CAD build for the part. Positions are in the model's coordinates, mm. A direction names the side the tool comes from. Coordinates: 2 decimals unless noted, no trailing zeros. Write each loop counter-clockwise with the first axis right and the second up, starting at its lowest first coordinate (ties: lowest second). Pieces come first, ordered by that corner, then holes. Notation, with made-up numbers: (-38.5, -20.5) -> (-9.5, -20.5) arc R22 cw to (-9.5, -8.5) -> close; hole circle Ø2 at (-25.75, 49.25). An arc over 180 degrees is marked (long way). Answer as CSV lines item,"result".
```python
from build123d import *

# Parameters (mm, degrees)
SKETCH1_W           = 12.7
SKETCH1_H           = 2.54
SKETCH1_W_2         = 1.27
SKETCH1_H_2         = 1.27
BOSS_EXTRUDE1_DEPTH = 2.54


with BuildPart() as part:
    # Sketch1 → Boss-Extrude1 (new body)
    with BuildSketch(Plane(origin=(0, 0, 0), x_dir=(1, 0, 0), z_dir=(0, 1, 0))):
        with Locations((6.35, 1.27)):
            Rectangle(SKETCH1_W, SKETCH1_H)
        with Locations((3.81, 1.27)):
            Rectangle(SKETCH1_W_2, SKETCH1_H_2, mode=Mode.SUBTRACT)
        with Locations((1.27, 1.27)):
            Rectangle(SKETCH1_W_2, SKETCH1_H_2, mode=Mode.SUBTRACT)
        with Locations((6.35, 1.27)):
            Rectangle(SKETCH1_W_2, SKETCH1_H_2, mode=Mode.SUBTRACT)
        with Locations((8.89, 1.27)):
            Rectangle(SKETCH1_W_2, SKETCH1_H_2, mode=Mode.SUBTRACT)
        with Locations((11.43, 1.27)):
            Rectangle(SKETCH1_W_2, SKETCH1_H_2, mode=Mode.SUBTRACT)
    extrude(amount=BOSS_EXTRUDE1_DEPTH)


solid = part.part
```
Item 1: Saw through at C-C on x = 6.5. Give the cut face in (y, z) (3 decimals).
Answer below:
outline,"(0, -2.54) -> (2.54, -2.54) -> (2.54, -1.905) -> (0, -1.905) -> close; (0, -0.635) -> (2.54, -0.635) -> (2.54, 0) -> (0, 0) -> close"
Item 2: Saw through at A-A on z = -1.3. Give the cut face in (x, y) (3 decimals).
Answer below:
outline,"(0, 0) -> (0.635, 0) -> (0.635, 2.54) -> (0, 2.54) -> close; (1.905, 0) -> (3.175, 0) -> (3.175, 2.54) -> (1.905, 2.54) -> close; (4.445, 0) -> (5.715, 0) -> (5.715, 2.54) -> (4.445, 2.54) -> close; (6.985, 0) -> (8.255, 0) -> (8.255, 2.54) -> (6.985, 2.54) -> close; (9.525, 0) -> (10.795, 0) -> (10.795, 2.54) -> (9.525, 2.54) -> close; (12.065, 0) -> (12.7, 0) -> (12.7, 2.54) -> (12.065, 2.54) -> close"
Item 3: Two-plate mould, pull along X, no slides. Class faces 1 (the flat face through (6, 1, -2.54)), 2 (the flat face through (0, 1, -1)), 3 (the flat face through (1, 1, -1.905)), 4 (the flat face through (9.525, 1, -1)): pulls with the +X half, pulls with the -X half, needs draft (parallel to the pull), parting line crosses it, or undercut.
Answer below:
face 1,"needs draft"
face 2,"pulls with the -X half"
face 3,"undercut"
face 4,"undercut"
Item 4: Saw through at B-B on y = 1.95. Give the cut face in (x, z) (3 decimals).
Answer below:
outline,"(0, -2.54) -> (12.7, -2.54) -> (12.7, 0) -> (0, 0) -> close; hole (0.635, -1.905) -> (1.905, -1.905) -> (1.905, -0.635) -> (0.635, -0.635) -> close; hole (3.175, -1.905) -> (4.445, -1.905) -> (4.445, -0.635) -> (3.175, -0.635) -> close; hole (5.715, -1.905) -> (6.985, -1.905) -> (6.985, -0.635) -> (5.715, -0.635) -> close; hole (8.255, -1.905) -> (9.525, -1.905) -> (9.525, -0.635) -> (8.255, -0.635) -> close; hole (10.795, -1.905) -> (12.065, -1.905) -> (12.065, -0.635) -> (10.795, -0.635) -> close"
Item 5: Wall check: line 1 (X direction, y = 0.75, z = -1.4) (3 decimals); line 2 (Z direction, x = 6, y = 1) (3 decimals). Give the ranges that are in metal, low to high. Write a range as from..to.
Answer below:
line 1,"x = 0..0.635, 1.905..3.175, 4.445..5.715, 6.985..8.255, 9.525..10.795, 12.065..12.7"
line 2,"z = -2.54..-1.905, -0.635..0"
Item 6: Flat gauge pin, fed straight in: pin 1 (1.4 mm diameter, centred on y = 2, z = -1, fed in from -X). Where does the tip first touch, or does it go through?
Answer below:
pin 1,"stops at x = 0"
Item 7: 3-axis set-ups, long thin cutter, end or side, ignore diameter. For faces 5 (the flat face through (5.715, 1, -1)), 6 (the flat face through (5, 2.54, -1)): which of +Z, -Z, +X, -X, +Y, -Y reach the whole face in a straight line?
Answer below:
face 5,"+Y, -Y"
face 6,"+Z, -Z, +X, -X, +Y"
